Read the model definition and answer for the solid it produces. Units are mm, in the model's axes. A direction names the side the tool comes from. Coordinates: 2 decimals unless noted, no trailing zeros. Loops run counter-clockwise (first coordinate to the right, second up) from the corner with the lowest first, then second, coordinate; pieces in that order, holes last. Notation, with made-up numbers: (66.25, -39.5) - (101.25, -39.5) arc R10 cw to (101.25, -29.5) - close; hole circle Ø5 at (11.25, -18). An arc over 180 degrees is marked (long way). One line per question, with ' | ' between items. Start each with the question number.
```python
from build123d import *

# Parameters (mm, degrees)
SKETCH1_W           = 30
SKETCH1_H           = 60
BOSS_EXTRUDE1_DEPTH = 3
BOSS_EXTRUDE2_START = -12
SKETCH2_R           = 4
BOSS_EXTRUDE2_DEPTH = 12
SKETCH8_R           = 2.5
CUT_EXTRUDE1_DEPTH  = 4
CHAMFER1_SIZE       = 1
CHAMFER1_SIZE2      = 2


with BuildPart() as part:
    # Sketch1 → Boss-Extrude1 (new body)
    with BuildSketch(Plane(origin=(0, 0, 0), x_dir=(1, 0, 0), z_dir=(0, 1, 0))):
        Rectangle(SKETCH1_W, SKETCH1_H)
    extrude(amount=BOSS_EXTRUDE1_DEPTH)

    # Sketch2 → Boss-Extrude2 (add)
    with BuildSketch(Plane.XY.offset(30).offset(BOSS_EXTRUDE2_START)):
        with BuildLine():
            Line((-15, 0), (-20, 0))
            ThreePointArc((-20, 0), (-17.5, 12.735742832), (-15, 0))
        make_face()
        with Locations((-17.5, 6.122498999)):
            Circle(SKETCH2_R, mode=Mode.SUBTRACT)
    boss_extrude2 = extrude(amount=-BOSS_EXTRUDE2_DEPTH)

    # Mirror1: Boss-Extrude2 across plane
    add(boss_extrude2.mirror(Plane.XY))

    # Sketch8 → Cut-Extrude1 (cut, through all)
    with BuildSketch(Plane(origin=(0, 3, 0), x_dir=(1, 0, 0), z_dir=(0, 1, 0))):
        with Locations((7.5, -18)):
            Circle(SKETCH8_R)
        with Locations((-7.5, -6)):
            Circle(SKETCH8_R)
        with Locations((7.5, 6)):
            Circle(SKETCH8_R)
        with Locations((-7.5, 18)):
            Circle(SKETCH8_R)
    extrude(amount=-CUT_EXTRUDE1_DEPTH, mode=Mode.SUBTRACT)

    # Chamfer1
    chamfer1_edges = [part.edges().sort_by_distance(p)[0] for p in [
        (-10, 3, -18),
        (-10, 3, 6),
        (5, 3, 18),
        (5, 3, -6),
    ]]
    chamfer1_side = [part.faces().sort_by_distance(p)[0] for p in [
        (0.649167265, 3, 0),
    ]]
    chamfer(chamfer1_edges, length=CHAMFER1_SIZE, length2=CHAMFER1_SIZE2, reference=chamfer1_side[0])


solid = part.part
```
1) The part is cut by section A-A on x = -7.5. Write down the section's boundary in (y, z), and give its area (3 significant figures).
2) The part is cut by section C-C on y = 4.5. Write down the section's boundary in (x, z).
3) Find the intervals of material crossed by line 1 along Z through (x, y) = (7.5, 0.45); line 2 along Y through (x, z) = (-17.5, -13.25); line 3 along Z through (x, y) = (-21, 10.25), in increasing order. Write a range as from..to.
4) Which of the six approach directions +Z, -Z, +X, -X, +Y, -Y give full straight-line access (tool end or side, diameter ignored) to faces 1 (the flat face through (0, 1, 30)), 2 (the flat face through (-20.3, 9.3, 6)), 3 (the flat face through (-20.3, 9.3, 18)), 4 (the flat face through (-20.3, 9.3, -18))?
5) The part is cut by section D-D on z = -7.5. Count the separate pieces of the cut face and the enclosed holes in it, and give its area (3 significant figures).
6) Given pin 1 Ø3 at (x, y) = (-17.5, 4) entering from +Z; pin 2 Ø3.5 at (y, z) = (2, -2.5) entering from -X; pin 3 Ø4 at (x, y) = (-14.5, 5.5) entering from +Z; pin 4 Ø6.5 at (x, z) = (-7.5, -18) entering from +Y, each flat-ended and moving along its own axis, determine where each tip first touches the part or whether it passes through.
7) The mould has two halves that part along Z. Classify faces 5 (the cylindrical face through (-20.674, 3.689, -12.084)), 6 (the flat face through (0, 1, -30)), 7 (the flat face through (-20.3, 9.3, -6)): released by +Z, released by -Z, zero draft, split by the parting line, or undercut.
8) The part is cut by section B-B on x = -17.5. Write down the section's boundary in (y, z).
Answer below:
1) outline: (0, -30) - (3, -30) - (3, -21.5) - (1, -20.5) - (0, -20.5) - close; (0, -15.5) - (1, -15.5) - (3, -14.5) - (3, 2.5) - (1, 3.5) - (0, 3.5) - close; (0, 8.5) - (1, 8.5) - (3, 9.5) - (3, 30) - (0, 30) - close | area: 146 mm2
2) outline: (-23.91, -18) - (-21.16, -18) - (-21.16, -6) - (-23.91, -6) - close; (-23.91, 6) - (-21.16, 6) - (-21.16, 18) - (-23.91, 18) - close; (-13.84, -18) - (-11.09, -18) - (-11.09, -6) - (-13.84, -6) - close; (-13.84, 6) - (-11.09, 6) - (-11.09, 18) - (-13.84, 18) - close
3) line 1: -30..-8.5, -3.5..15.5, 20.5..30 | line 2: 0..2.12, 10.12..12.74 | line 3: -18..-6, 6..18
4) face 1: +Z, +X, -X, +Y, -Y | face 2: -X, +Y | face 3: +Z, -X, +Y | face 4: -Z, -X, +Y
5) separate pieces: 2 | enclosed holes: 1 | area: 155 mm2
6) pin 1: through | pin 2: x = -15 | pin 3: z = 18 | pin 4: y = 2.5
7) face 5: zero draft | face 6: released by -Z | face 7: undercut
8) outline: (0, -18) - (2.12, -18) - (2.12, -6) - (0, -6) - close; (0, 6) - (2.12, 6) - (2.12, 18) - (0, 18) - close; (10.12, -18) - (12.74, -18) - (12.74, -6) - (10.12, -6) - close; (10.12, 6) - (12.74, 6) - (12.74, 18) - (10.12, 18) - close
